Could you check a few things on this model? Use its own coordinates, in mm. Face numbers are marked on the shaded views. A direction names the side the tool comes from. Coordinates: 2 decimals unless noted, no trailing zeros. Write each loop counter-clockwise with the first axis right and the second up, starting at its lowest first coordinate (ties: lowest second). Pieces come first, ordered by that corner, then holes. Notation, with made-up numbers: (66.25, -19) - (106.25, -19) arc R18 cw to (106.25, 11) - close; hole circle Ø3 at (57.25, -1.5). An arc over 180 degrees is marked (long way). Answer as a JSON object with one key per item and string values. Group by question number.
1) If we section it at B-B (y = 4.75): Write out the boundary of the cut face in (x, z).
2) Please list where these lines run through material, in increasing order: line 1 along Y through (x, z) = (11.5, 8); line 2 along Y through (x, z) = (8.25, -0.5); line 3 along Y through (x, z) = (5.25, 7).
3) If we section it at C-C (x = 3): Write out the boundary of the cut face in (y, z), plus the area to 3 significant figures.
4) Will these pins go through, and if not, where does the flat tip stop? pin 1 Ø1.6 at (x, z) = (10.5, -0.5) entering from -Y; pin 2 Ø3 at (x, y) = (1, -11) entering from -Z; pin 3 Ø1.6 at (x, z) = (-11, 2.5) entering from +Y.
5) If we section it at D-D (x = -2): Write out the boundary of the cut face in (y, z), plus the area to 3 significant figures.
6) We'd pull the mould along Y, two halves only. Please class the marked faces 6, 7 and 8: released by +Y, released by -Y, zero draft, split by the parting line, or undercut.
7) On a 3-axis mill with a long thin cutter (end or side, diameter ignored), from which of +Z, -Z, +X, -X, +Y, -Y can I reach the whole of each face in a straight line? I mean the marked faces 1, 2, 3, 4 and 5. Say none if no direction works.
8) If we section it at A-A (z = -0.5): Write out the boundary of the cut face in (x, y), plus the area to 3 significant figures.
```python
from build123d import *

# Parameters (mm, degrees)
SKETCH1_W           = 22
SKETCH1_H           = 22
BOSS_EXTRUDE1_DEPTH = 10
SKETCH3_W           = 2
SKETCH3_H           = 10
BOSS_EXTRUDE2_DEPTH = 2
SKETCH4_W           = 10
SKETCH4_H           = 2
BOSS_EXTRUDE3_DEPTH = 2
SKETCH5_W           = 10
SKETCH5_H           = 2
CUT_EXTRUDE1_DEPTH  = 2
SKETCH6_W           = 2
SKETCH6_H           = 10
CUT_EXTRUDE2_DEPTH  = 2
SKETCH7_R           = 9.2
CUT_EXTRUDE3_DEPTH  = 11
SKETCH8_W           = 6.75
SKETCH8_H           = 6.75
BOSS_EXTRUDE4_DEPTH = 2


with BuildPart() as part:
    # Sketch1 → Boss-Extrude1 (new body)
    with BuildSketch(Plane.XY):
        with Locations((1.600938967, -1.755868545)):
            Rectangle(SKETCH1_W, SKETCH1_H)
    extrude(amount=BOSS_EXTRUDE1_DEPTH)

    # Sketch3 → Boss-Extrude2 (add)
    with BuildSketch(Plane.XZ.offset(12.755868545)):
        with Locations((7.600938967, 5)):
            Rectangle(SKETCH3_W, SKETCH3_H)
        with Locations((-4.399061033, 5)):
            Rectangle(SKETCH3_W, SKETCH3_H)
    extrude(amount=BOSS_EXTRUDE2_DEPTH)

    # Sketch4 → Boss-Extrude3 (add)
    with BuildSketch(Plane.ZY.offset(9.399061033)):
        with Locations((5, 4.244131455)):
            Rectangle(SKETCH4_W, SKETCH4_H)
        with Locations((5, -7.755868545)):
            Rectangle(SKETCH4_W, SKETCH4_H)
    extrude(amount=BOSS_EXTRUDE3_DEPTH)

    # Sketch5 → Cut-Extrude1 (cut)
    with BuildSketch(Plane(origin=(12.600938967, 0, 0), x_dir=(0, 0, -1), z_dir=(1, 0, 0))):
        with Locations((-5, 4.244131455)):
            Rectangle(SKETCH5_W, SKETCH5_H)
        with Locations((-5, -7.755868545)):
            Rectangle(SKETCH5_W, SKETCH5_H)
    extrude(amount=-CUT_EXTRUDE1_DEPTH, mode=Mode.SUBTRACT)

    # Sketch6 → Cut-Extrude2 (cut)
    with BuildSketch(Plane(origin=(0, 9.244131455, 0), x_dir=(1, 0, 0), z_dir=(0, 1, 0))):
        with Locations((-4.399061033, -5)):
            Rectangle(SKETCH6_W, SKETCH6_H)
        with Locations((7.600938967, -5)):
            Rectangle(SKETCH6_W, SKETCH6_H)
    extrude(amount=-CUT_EXTRUDE2_DEPTH, mode=Mode.SUBTRACT)

    # Sketch7 → Cut-Extrude3 (cut, through all)
    with BuildSketch(Plane.XY.offset(10)):
        with Locations((1.600938967, -1.755868545)):
            Circle(SKETCH7_R)
    extrude(amount=-CUT_EXTRUDE3_DEPTH, mode=Mode.SUBTRACT)

    # Sketch8 → Boss-Extrude4 (add)
    with BuildSketch(Plane(origin=(0, 0, 0), x_dir=(-1, 0, 0), z_dir=(0, 0, -1))):
        with Locations((6.024061033, 5.869131455)):
            Rectangle(SKETCH8_W, SKETCH8_H)
        with Locations((-9.225938967, 5.869131455)):
            Rectangle(SKETCH8_W, SKETCH8_H)
        with Locations((-9.225938967, -9.380868545)):
            Rectangle(SKETCH8_W, SKETCH8_H)
        with Locations((6.024061033, -9.380868545)):
            Rectangle(SKETCH8_W, SKETCH8_H)
    extrude(amount=BOSS_EXTRUDE4_DEPTH)


solid = part.part
```
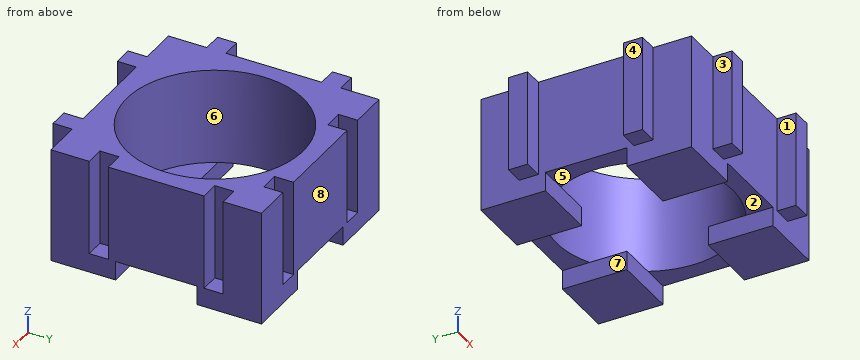
Here are the results:
{
 "1": {"outline": "(-11.4, 0) - (-9.4, 0) - (-9.4, -2) - (-2.65, -2) - (-2.65, 0) - (-4.9, 0) - (-4.9, 10) - (-11.4, 10) - close; (5.85, -2) - (12.6, -2) - (12.6, 0) - (10.6, 0) - (10.6, 10) - (8.11, 10) - (8.11, 0) - (5.85, 0) - close"},
 "2": {"line 1": "y = -12.76 to -8.76, -6.76 to 3.24, 5.24 to 9.24", "line 2": "y = -12.76 to -6.01, 2.49 to 9.24", "line 3": "y = -12.76 to -10.2, 6.69 to 9.24"},
 "3": {"outline": "(-12.76, 0) - (-10.85, 0) - (-10.85, 10) - (-12.76, 10) - close; (7.34, 0) - (9.24, 0) - (9.24, 10) - (7.34, 10) - close", "area": "38.1 mm²"},
 "4": {"pin 1": "stops at y = -12.76", "pin 2": "stops at z = 0", "pin 3": "stops at y = 5.24"},
 "5": {"outline": "(-12.76, 0) - (-10.22, 0) - (-10.22, 10) - (-12.76, 10) - close; (6.71, 0) - (9.24, 0) - (9.24, 10) - (6.71, 10) - close", "area": "50.7 mm²"},
 "6": {"face 6": "undercut", "face 7": "zero draft", "face 8": "released by +Y"},
 "7": {"face 1": "+Z, -Z, -Y", "face 2": "-Z, +Y, -Y", "face 3": "+Z, -Z, -X, -Y", "face 4": "+Z, -Z, -X, +Y, -Y", "face 5": "-Z, +X, -X"},
 "8": {"outline": "(-9.4, -12.76) - (-2.65, -12.76) - (-2.65, -6.01) - (-9.4, -6.01) - close; (-9.4, 2.49) - (-2.65, 2.49) - (-2.65, 9.24) - (-9.4, 9.24) - close; (5.85, -12.76) - (12.6, -12.76) - (12.6, -6.01) - (5.85, -6.01) - close; (5.85, 2.49) - (12.6, 2.49) - (12.6, 9.24) - (5.85, 9.24) - close", "area": "182 mm²"}
}
